from build123d import *

# Parameters (mm, degrees)
BOSS_EXTRUDE1_DEPTH = 1.524
SKETCH3_W           = 1.524
SKETCH3_H           = 1.524
CUT_EXTRUDE1_DEPTH  = 0.762


with BuildPart() as part:
    # Sketch1 → Boss-Extrude1 (new body)
    with BuildSketch(Plane.XY):
        Polygon((57.718435694, 0), (57.718435694, -1.524), (54.412176394, -1.524), (54.412176394, -2.617357602), (56.936958373, -2.617357602), (59.461740351, -4.787750638), (60.985740351, -4.787750638), (60.985740351, -3.263750638), (59.461740351, -3.263750638), (59.461740351, 1.739750638), (60.985740351, 1.739750638), (60.985740351, 3.263750638), (59.461740351, 3.263750638), (56.936958373, 1.093357602), (54.412176394, 1.093357602), (54.412176394, 0), align=None)
    extrude(amount=BOSS_EXTRUDE1_DEPTH)

    # Sketch3 → Cut-Extrude1 (cut)
    with BuildSketch(Plane(origin=(0, 1.093357602, 0), x_dir=(1, 0, 0), z_dir=(0, 1, 0))):
        with Locations((55.682176394, -0.762)):
            Rectangle(SKETCH3_W, SKETCH3_H)
    cut_extrude1 = extrude(amount=-CUT_EXTRUDE1_DEPTH, mode=Mode.SUBTRACT)

    # Mirror1: Cut-Extrude1 across plane
    add(cut_extrude1.mirror(Plane.ZX.offset(-0.762)), mode=Mode.SUBTRACT)


solid = part.part
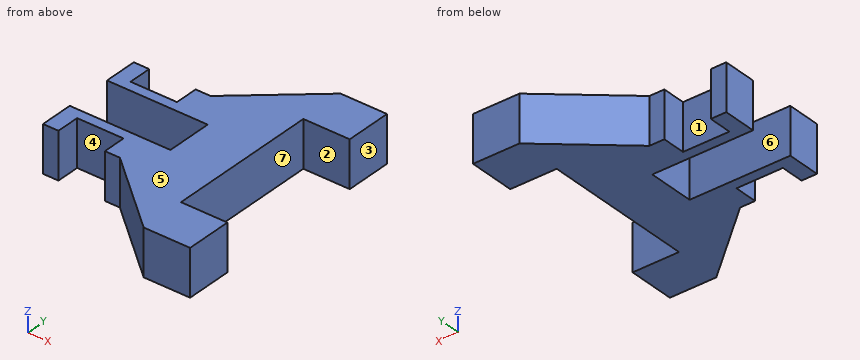
Could you check a few things on this model? Use its own coordinates, in mm. Face numbers are marked on the shaded views. A direction names the side the tool comes from. Give positions to 0.01 mm unless a question says otherwise; leave off trailing zeros. Order: outer loops, then holes, each group sorted by start corner. A loop starts at its lowest first (then second) coordinate and runs counter-clockwise, first axis right, second up.
Item 1: If we section it at C-C, the plane z = 0.45: Write out the boundary of the cut face in (x, y).
Item 2: If we mould it in two halves opening along Y, with no side actions, what happens to the marked faces 1, 2 and 3? For each: pulls with the +Y half, pulls with the -Y half, needs draft (parallel to the pull), parting line crosses it, or undercut.
Item 3: I'm going to push flat-ended pins straight in: pin 1 (0.5 mm diameter, centred on y = -1.5, z = 0.5, fed in from +X); pin 2 (0.8 mm diameter, centred on x = 55.5, z = 0.5, fed in from -Y); pin 3 (0.8 mm diameter, centred on y = -0.5, z = 0.5, fed in from -X); pin 4 (3 mm diameter, centred on x = 55.5, y = 1, fed in from -Z). Where does each tip first touch, or does it pass through?
Item 4: If we section it at D-D, the plane y = -3.5: Write out the boundary of the cut face in (x, z), plus the area to 3 significant figures.
Item 5: If we section it at A-A, the plane x = 56.25: Write out the boundary of the cut face in (y, z).
Item 6: I need wall thicknesses on line 1 (Y direction, x = 60, z = 0.2); line 2 (X direction, y = -2.25, z = 0.3); line 3 (Y direction, x = 55, z = 1.4). Which ranges of each line are inside material? Lowest first, please.
Item 7: If we section it at B-B, the plane y = -2.5: Write out the boundary of the cut face in (x, z), plus the area to 3 significant figures.
Item 8: For the marked faces 4, 5, 6 and 7, which set-ups out of +Z, -Z, +X, -X, +Y, -Y let a thin tool reach every point of the face, with its end or its side?
Values:
1. outline: (54.41, -2.62) - (54.92, -2.62) - (54.92, -1.86) - (56.44, -1.86) - (56.44, -2.62) - (56.94, -2.62) - (59.46, -4.79) - (60.99, -4.79) - (60.99, -3.26) - (59.46, -3.26) - (59.46, 1.74) - (60.99, 1.74) - (60.99, 3.26) - (59.46, 3.26) - (56.94, 1.09) - (56.44, 1.09) - (56.44, 0.33) - (54.92, 0.33) - (54.92, 1.09) - (54.41, 1.09) - (54.41, 0) - (57.72, 0) - (57.72, -1.52) - (54.41, -1.52) - close
2. face 1: pulls with the +Y half
2. face 2: undercut
2. face 3: needs draft
3. pin 1: stops at x = 59.46
3. pin 2: stops at y = -1.86
3. pin 3: stops at x = 57.72
3. pin 4: stops at z = 0
4. outline: (57.96, 0) - (60.99, 0) - (60.99, 1.52) - (57.96, 1.52) - close
4. area: 4.61 mm2
5. outline: (-1.86, 0) - (-1.52, 0) - (-1.52, 1.52) - (-1.86, 1.52) - close; (0, 0) - (0.33, 0) - (0.33, 1.52) - (0, 1.52) - close
6. line 1: y = -4.79 to -3.26, 1.74 to 3.26
6. line 2: x = 54.41 to 54.92, 56.44 to 59.46
6. line 3: y = -1.86 to -1.52, 0 to 0.33
7. outline: (54.41, 0) - (54.92, 0) - (54.92, 1.52) - (54.41, 1.52) - close; (56.44, 0) - (59.46, 0) - (59.46, 1.52) - (56.44, 1.52) - close
7. area: 5.37 mm2
8. face 4: +Z, -Z, -Y
8. face 5: +Z, +X, -X, +Y, -Y
8. face 6: +Z, -Z, -X
8. face 7: +Z, -Z, +X
